from build123d import *

# Parameters (mm, degrees)
F0_W      = 1245
F0_H      = 2585
F1_DEPTH  = 410
F2_T      = -10
F3_W      = 1225
F3_H      = 5
F4_DEPTH  = 400
F5_W      = 10
F5_H      = 672.5
F6_DEPTH  = 400
F7_W      = 915
F7_H      = 10
F8_DEPTH  = 400
F9_W      = 10
F9_H      = 300
F10_DEPTH = 400
F11_W     = 10
F11_H     = 336.25
F12_DEPTH = 400
F13_W     = 1225
F13_H     = 10
F14_DEPTH = 400
F15_W     = 10
F15_H     = 791.25
F16_DEPTH = 400
F17_W     = 612.5
F17_H     = 10
F18_DEPTH = 400
F19_W     = 10
F19_H     = 781.25
F20_DEPTH = 400
F21_W     = 865
F21_H     = 10
F22_DEPTH = 400


with BuildPart() as f1:
    # F0 (on Front) → F1 (new body)
    with BuildSketch(Plane.XZ):
        with Locations((622.5, 1292.5)):
            Rectangle(F0_W, F0_H)
    extrude(amount=F1_DEPTH)

    # F2
    f2_openings = [f1.faces().sort_by_distance(p)[0] for p in [
        (622.5, -410, 1292.5),
    ]]
    offset(amount=F2_T, openings=f2_openings)

    # F3 (on face) → F4 (join)
    with BuildSketch(Plane.XZ.offset(10)):
        with Locations((622.5, 2272.5)):
            Rectangle(F3_W, F3_H)
        with Locations((622.5, 1595)):
            Rectangle(F3_W, F3_H)
    extrude(amount=F4_DEPTH)

    # F5 (on face) → F6 (join)
    with BuildSketch(Plane.XZ.offset(10)):
        with Locations((315, 1933.75)):
            Rectangle(F5_W, F5_H)
    extrude(amount=F6_DEPTH)

    # F7 (on face) → F8 (join)
    with BuildSketch(Plane.XZ.offset(10)):
        with Locations((777.5, 1938.75)):
            Rectangle(F7_W, F7_H)
    extrude(amount=F8_DEPTH)

    # F9 (on face) → F10 (join)
    with BuildSketch(Plane.XZ.offset(10)):
        with Locations((630, 2425)):
            Rectangle(F9_W, F9_H)
    extrude(amount=F10_DEPTH)

    # F11 (on face) → F12 (join)
    with BuildSketch(Plane.XZ.offset(10)):
        with Locations((782.5, 1765.625)):
            Rectangle(F11_W, F11_H)
    extrude(amount=F12_DEPTH)

    # F13 (on face) → F14 (join)
    with BuildSketch(Plane.XZ.offset(10)):
        with Locations((622.5, 796.25)):
            Rectangle(F13_W, F13_H)
    extrude(amount=F14_DEPTH)

    # F15 (on face) → F16 (join)
    with BuildSketch(Plane.XZ.offset(10)):
        with Locations((627.5, 1196.875)):
            Rectangle(F15_W, F15_H)
    extrude(amount=F16_DEPTH)

    # F17 (on face) → F18 (join)
    with BuildSketch(Plane.XZ.offset(10)):
        with Locations((316.25, 1191.875)):
            Rectangle(F17_W, F17_H)
    extrude(amount=F18_DEPTH)

    # F19 (on face) → F20 (join)
    with BuildSketch(Plane.XZ.offset(10)):
        with Locations((880, 400.625)):
            Rectangle(F19_W, F19_H)
    extrude(amount=F20_DEPTH)

    # F21 (on face) → F22 (join)
    with BuildSketch(Plane.XZ.offset(10)):
        with Locations((442.5, 395.625)):
            Rectangle(F21_W, F21_H)
    extrude(amount=F22_DEPTH)


solid = f1.part
Can you work these out from the model? Positions are in its coordinate system, mm. Round coordinates to 2 decimals unless told otherwise and drop trailing zeros. Loops run counter-clockwise (first coordinate to the right, second up) from the corner with the lowest first, then second, coordinate; pieces in that order, holes last. Notation, with made-up numbers: (75.5, 20) - (117.5, 20) arc R22 ccw to (117.5, 51) - close; hole circle Ø11 at (52, 66). An arc over 180 degrees is marked (long way). Answer in a Markdown table with one row per item. Add a question column.
Q1. For pin 1 Ø3 at (x, z) = (655, 1534) entering from -Y, with a flat end and sliding along its axis, tell me the tip position at first contact or that it passes through.
Q2. I want a section at C-C on y = -345.5. Count the separate pieces of the cut face and the enclosed holes in it, and give its area (3 significant figures).
Q3. I want a section at D-D on x = 945. List the corners of the cut face in (y, z) for me, and give its area (4 significant figures).
Q4. I want a section at B-B on z = 1498.5. List the corners of the cut face in (x, y) for me, and give its area (4 significant figures).
Q5. I need wall thicknesses on L1, parallel to Z at x = 1151.5, y = -119; L2, parallel to X at y = -179, z = 1638; L3, parallel to X at y = -150, z = 129.5. Which ranges of each line are inside material? Lowest first, please.
A:
| question | item | result |
|---|---|---|
| 1 | pin 1 | y = -10 |
| 2 | separate pieces | 1 |
| 2 | enclosed holes | 12 |
| 2 | area | 153,000 mm^2 |
| 3 | outline | (-410, 0) - (0, 0) - (0, 2585) - (-410, 2585) - (-410, 2575) - (-10, 2575) - (-10, 2275) - (-410, 2275) - (-410, 2270) - (-10, 2270) - (-10, 1943.75) - (-410, 1943.75) - (-410, 1933.75) - (-10, 1933.75) - (-10, 1597.5) - (-410, 1597.5) - (-410, 1592.5) - (-10, 1592.5) - (-10, 801.25) - (-410, 801.25) - (-410, 791.25) - (-10, 791.25) - (-10, 10) - (-410, 10) - close |
| 3 | area | 45,850 mm^2 |
| 4 | outline | (0, -410) - (10, -410) - (10, -10) - (622.5, -10) - (622.5, -410) - (632.5, -410) - (632.5, -10) - (1235, -10) - (1235, -410) - (1245, -410) - (1245, 0) - (0, 0) - close |
| 4 | area | 24,450 mm^2 |
| 5 | L1 | 0 to 10, 791.25 to 801.25, 1592.5 to 1597.5, 1933.75 to 1943.75, 2270 to 2275, 2575 to 2585 |
| 5 | L2 | 0 to 10, 310 to 320, 777.5 to 787.5, 1235 to 1245 |
| 5 | L3 | 0 to 10, 875 to 885, 1235 to 1245 |
